```python
from build123d import *

# Parameters (mm, degrees)
SKETCH1_W           = 45
SKETCH1_H           = 50
BOSS_EXTRUDE1_DEPTH = 45
SKETCH2_R           = 5.2
CUT_EXTRUDE1_DEPTH  = 45
SKETCH3_R           = 19.125
CUT_EXTRUDE2_DEPTH  = 45
SKETCH4_W           = 12.5
SKETCH4_H           = 4.851403087
CUT_EXTRUDE3_DEPTH  = 45
SKETCH5_R           = 19.125
BOSS_EXTRUDE2_DEPTH = 6
SKETCH6_R           = 10.6
CUT_EXTRUDE4_DEPTH  = 6
SKETCH7_R           = 19.5
CUT_EXTRUDE5_DEPTH  = 39
SKETCH8_W           = 0.25
SKETCH8_H           = 2.013794316
BOSS_EXTRUDE3_DEPTH = 45
SKETCH9_R           = 5.15
CUT_EXTRUDE6_DEPTH  = 2
SKETCH10_R          = 5.15
CUT_EXTRUDE7_DEPTH  = 2


with BuildPart() as part:
    # Sketch1 → Boss-Extrude1 (new body)
    with BuildSketch(Plane.XY):
        with Locations((8.236607143, -2.901785714)):
            Rectangle(SKETCH1_W, SKETCH1_H)
    extrude(amount=BOSS_EXTRUDE1_DEPTH)

    # Sketch2 → Cut-Extrude1 (cut)
    with BuildSketch(Plane.XY.offset(45)):
        with Locations((-4.163392857, -24.901785714)):
            Circle(SKETCH2_R)
        with Locations((20.636607143, -24.901785714)):
            Circle(SKETCH2_R)
    extrude(amount=-CUT_EXTRUDE1_DEPTH, mode=Mode.SUBTRACT)

    # Sketch3 → Cut-Extrude2 (cut)
    with BuildSketch(Plane(origin=(30.736607143, 0, 0), x_dir=(0, 0, -1), z_dir=(1, 0, 0))):
        with Locations((-22.5, 1.613158508)):
            Circle(SKETCH3_R)
    extrude(amount=-CUT_EXTRUDE2_DEPTH, mode=Mode.SUBTRACT)

    # Sketch4 → Cut-Extrude3 (cut)
    with BuildSketch(Plane(origin=(30.736607143, 0, 0), x_dir=(0, 0, -1), z_dir=(1, 0, 0))):
        with Locations((-22.5, 20.946020309)):
            Rectangle(SKETCH4_W, SKETCH4_H)
    extrude(amount=-CUT_EXTRUDE3_DEPTH, mode=Mode.SUBTRACT)

    # Sketch5 → Boss-Extrude2 (add)
    with BuildSketch(Plane(origin=(30.736607143, 0, 0), x_dir=(0, 0, -1), z_dir=(1, 0, 0))):
        with Locations((-22.5, 1.613158508)):
            Circle(SKETCH5_R)
    extrude(amount=-BOSS_EXTRUDE2_DEPTH)

    # Sketch6 → Cut-Extrude4 (cut)
    with BuildSketch(Plane(origin=(30.736607143, 0, 0), x_dir=(0, 0, -1), z_dir=(1, 0, 0))):
        with Locations((-22.5, 1.613158508)):
            Circle(SKETCH6_R)
    extrude(amount=-CUT_EXTRUDE4_DEPTH, mode=Mode.SUBTRACT)

    # Sketch7 → Cut-Extrude5 (cut)
    with BuildSketch(Plane.ZY.offset(14.263392857)):
        with Locations((22.5, 1.613158508)):
            Circle(SKETCH7_R)
    extrude(amount=-CUT_EXTRUDE5_DEPTH, mode=Mode.SUBTRACT)

    # Sketch8 → Boss-Extrude3 (add)
    with BuildSketch(Plane.ZY.offset(14.263392857)):
        with Locations((16.375, 21.091317128)):
            Rectangle(SKETCH8_W, SKETCH8_H)
        with Locations((28.625, 21.091317128)):
            Rectangle(SKETCH8_W, SKETCH8_H)
    extrude(amount=-BOSS_EXTRUDE3_DEPTH)

    # Sketch9 → Cut-Extrude6 (cut)
    with BuildSketch(Plane.XY.offset(45)):
        with Locations((8.236607143, -2.401785714)):
            Circle(SKETCH9_R)
    extrude(amount=-CUT_EXTRUDE6_DEPTH, mode=Mode.SUBTRACT)

    # Sketch10 → Cut-Extrude7 (cut)
    with BuildSketch(Plane(origin=(0, 0, 0), x_dir=(-1, 0, 0), z_dir=(0, 0, -1))):
        with Locations((-8.236607143, -2.401785714)):
            Circle(SKETCH10_R)
    extrude(amount=-CUT_EXTRUDE7_DEPTH, mode=Mode.SUBTRACT)


solid = part.part
```
The model under review builds one solid part; all positions refer to its coordinate system, in mm. A direction names the side the tool comes from. Give positions to 0.01 mm unless a question says otherwise; leave off trailing zeros. Write each loop counter-clockwise with the first axis right and the second up, starting at its lowest first coordinate (ties: lowest second). Pieces come first, ordered by that corner, then holes. Notation, with made-up numbers: M -27,31 L 13,31 A17 cw 13,50 Z; hole C -27.5,-38.5 d6. An arc over 180 degrees is marked long. Write each question's results on one line, items separated by ' | '. Start each with the question number.
1. We need section C-C (y = 11). Write out the cut boundary in (x, z), and give its area (3 significant figures).
2. Insertion check: pin 1 Ø11.5 at (x, y) = (6, -3.5) entering from +Z; pin 2 Ø8 at (x, y) = (8.24, -2.4) entering from -Z; pin 3 Ø3 at (x, z) = (18.5, 23.5) entering from -Y; pin 4 Ø2 at (y, z) = (-4, 9.5) entering from -X. Each pin has a flat end and moves straight along its axis. Give the tip position at first contact, or say it passes through.
3. For probe 1 along X at (y, z) = (-26, 7.5); probe 2 along X at (y, z) = (11, 6); probe 3 along Z at (x, y) = (24.5, 19.5), list the stretches that pass through material, from the lowest coordinate up. Write a range as [from, to].
4. Mouldability with a two-part tool opening along Z and no side actions: class faces 6 (the flat face through (8, 21, 16.5)), 7 (the flat face through (8, -2, 43)), 8 (the flat face through (8, -2, 2)), 9 (the cylindrical face through (20.796, -19.704, 22.815)) as released by +Z, released by -Z, zero draft, split by the parting line, or undercut.
5. For faces 1 (the flat face through (28, -27.902, 22)), 2 (the cylindrical face through (4.44, 1.08, 44.01)), 3 (the flat face through (24.737, -7, 14)), 4 (the cylindrical face through (3.324, -0.855, 0.986)), 5 (the flat face through (8, 22.098, 37)), list the 3-axis set-ups (+Z, -Z, +X, -X, +Y, -Y) from which the entire face can be reached by the end or side of a thin tool; tool diameter is ignored.
6. We need section B-B (x = 27). Write out the cut boundary in (y, z) (3 decimals), and give its area (3 significant figures).
7. We need section D-D (x = -4). Write out the cut boundary in (y, z).
8. We need section A-A (z = 22.5). Write out the cut boundary in (x, y).
Results found:
1) outline: M -14.26,0 L 30.74,0 L 30.74,17.58 L 24.74,17.58 L 24.74,5.41 L -14.26,5.41 Z; M -14.26,39.59 L 24.74,39.59 L 24.74,27.42 L 30.74,27.42 L 30.74,45 L -14.26,45 Z | area: 633 mm^2
2) pin 1: stops at z = 45 | pin 2: stops at z = 2 | pin 3: stops at y = -21.18 | pin 4: stops at x = 24.74
3) probe 1: x = [-14.26, -9.25], [0.92, 15.55], [25.72, 30.74] | probe 2: x = [24.74, 30.74] | probe 3: z = [0, 14.73], [30.27, 45]
4) face 6: undercut | face 7: released by +Z | face 8: released by -Z | face 9: zero draft
5) face 1: +Z, -Z, +X, -X, -Y | face 2: +Z | face 3: -X | face 4: -Z | face 5: +Z, -Z, +X, -X, +Y
6) outline: M -27.902,0 L 22.098,0 L 22.098,16.5 L 20.084,16.5 L 20.084,16.25 L 19.688,16.25 A19.125 ccw 19.688,28.75 L 20.084,28.75 L 20.084,28.5 L 22.098,28.5 L 22.098,45 L -27.902,45 Z; hole C 1.613,22.5 d21.2 | area: 1,880 mm^2
7) outline: M -19.7,0 L 22.1,0 L 22.1,16.5 L 20.08,16.5 L 20.08,16.25 A19.5 cw long 20.08,28.75 L 20.08,28.5 L 22.1,28.5 L 22.1,45 L -19.7,45 Z
8) outline: M -14.26,-27.9 L -8.41,-27.9 A5.2 cw long 0.08,-27.9 L 16.39,-27.9 A5.2 cw long 24.88,-27.9 L 30.74,-27.9 L 30.74,-8.99 L 24.74,-8.99 L 24.74,-17.89 L -14.26,-17.89 Z; M 24.74,12.21 L 30.74,12.21 L 30.74,20.74 L 24.74,20.74 Z
